Geometry: final body of the model. Coordinates: model frame, mm. Face numbers are marked on the shaded views. A direction names the side the tool comes from. Coordinates: 2 decimals unless noted, no trailing zeros. Write each loop counter-clockwise with the first axis right and the second up, starting at its lowest first coordinate (ties: lowest second). Pieces come first, ordered by that corner, then holes. Notation, with made-up numbers: M 12.25,-0.75 L 64.25,-0.75 A10 ccw 64.25,13.25 Z; hole C 58,84.5 d6. An arc over 180 degrees is marked long. Write item = value, one per line. Start each with the question number.
Item 1: Section C-C on x = 0. Output: boundary loops of the cut face in (y, z).
Item 2: Ray query, L1, parallel to X at y = -11.5, z = 0; L2, parallel to X at y = -4.5, z = 14; L3, parallel to Z at x = 0, y = -32.5. Return the intervals inside material, ascending. Write a range as [from, to].
Item 3: Reachability of the marked faces 4, 5, 6, 7 and 8 from +Z, -Z, +X, -X, +Y, -Y: full face, straight path, thin tool, end or side. Return the list, or none.
Item 4: Section A-A on z = 0. Output: boundary loops of the cut face in (x, y), plus the area to 3 significant figures.
Item 5: Section D-D on z = 19.5. Output: boundary loops of the cut face in (x, y).
Item 6: Pull-direction query (X, two-part tool) for the marked faces 1, 2 and 3; classes: +X half, -X half, draft (parallel to the pull), parting line (faces both ways), or undercut.
Item 7: Section B-B on y = -32.15. Output: boundary loops of the cut face in (x, z).
Item 8: First-contact query: pin 1 Ø5 at (x, z) = (-3.5, 13) entering from -Y; pin 2 Ø17 at (y, z) = (-13, 26.5) entering from +X; pin 3 Ø2 at (x, y) = (9.5, 6.5) entering from -Z; pin 4 Ø1.5 at (x, y) = (10, -40) entering from -Z. Flat tips, straight axial feed; report the tip coordinate or a pass-through.
from build123d import *

# Parameters (mm, degrees)
F0_R     = 13.25
F1_DEPTH = 50
F2_R     = 9.65
F3_DEPTH = 30.301
F5_DEPTH = 30.301
F7_DEPTH = 27.7
F8_W     = 11.7
F8_H     = 11.66135
F9_DEPTH = 50.001


with BuildPart() as f1:
    # F0 (on Front) → F1 (new body)
    with BuildSketch(Plane.XZ):
        with BuildLine():
            Line((-13.85, 42.55), (-13.85, 8.87581))
            ThreePointArc((-13.85, 8.87581), (0, -16.45), (13.85, 8.87581))
            Line((13.85, 8.87581), (13.85, 42.55))
            Line((13.85, 42.55), (-13.85, 42.55))
        make_face()
        Circle(F0_R, mode=Mode.SUBTRACT)
    extrude(amount=F1_DEPTH)

    # F2 (on face) → F3 (cut, through all)
    with BuildSketch(Plane(origin=(-13.85, 0, 0), x_dir=(0, -1, 0), z_dir=(-1, 0, 0))):
        with Locations((32.15, 27.4)):
            Circle(F2_R)
    extrude(amount=-F3_DEPTH, mode=Mode.SUBTRACT)

    # F4 (on face) → F5 (cut, through all)
    with BuildSketch(Plane(origin=(-13.85, 0, 0), x_dir=(0, -1, 0), z_dir=(-1, 0, 0))):
        Polygon((0, 23.55), (6, 30.757681), (0, 34.363233), align=None)
    extrude(amount=-F5_DEPTH, mode=Mode.SUBTRACT)

    # F6 (on face) → F7 (join)
    with BuildSketch(Plane(origin=(-13.85, 0, 0), x_dir=(0, -1, 0), z_dir=(-1, 0, 0))):
        Polygon((-14.600857, 42.55), (0, 34.363233), (0, 42.55), align=None)
    extrude(amount=-F7_DEPTH)

    # F8 (on face) → F9 (cut, through all)
    with BuildSketch(Plane(origin=(0, 0, 0), x_dir=(-1, 0, 0), z_dir=(0, 1, 0))):
        with Locations((0, 17.719325)):
            Rectangle(F8_W, F8_H)
        with BuildLine():
            ThreePointArc((13.25, 0), (11.248889, 7.001785), (5.85, 11.88865))
            Line((5.85, 11.88865), (-5.85, 11.88865))
            ThreePointArc((-5.85, 11.88865), (-7.001785, -11.248889), (13.25, 0))
        make_face()
    extrude(amount=-F9_DEPTH, mode=Mode.SUBTRACT)


solid = f1.part
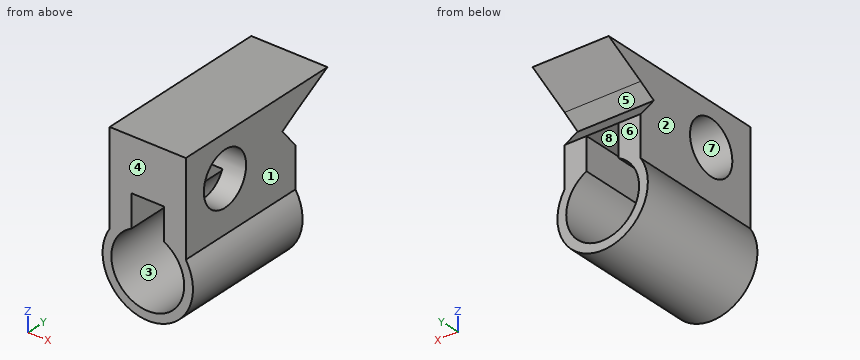
Responses:
q1.outline = M -50,-16.45 L 0,-16.45 L 0,-13.25 L -50,-13.25 Z; M -50,23.55 L -41,23.55 A9.65 cw long -23.3,23.55 L 0,23.55 L -6,30.76 L 0,34.36 L 14.6,42.55 L -50,42.55 Z
q2.L1 = [-16.45, -13.25], [13.25, 16.45]
q2.L2 = [-13.85, -5.85], [5.85, 13.85]
q2.L3 = [-16.45, -13.25], [37.04, 42.55]
q3.face_4 = +Z, -Z, +X, -X, -Y
q3.face_5 = +X, -X, +Y
q3.face_6 = -Z, +X, -X, +Y
q3.face_7 = +X, -X
q3.face_8 = +Y, -Y
q4.outline = M -16.45,-50 L -13.25,-50 L -13.25,0 L -16.45,0 Z; M 13.25,-50 L 16.45,-50 L 16.45,0 L 13.25,0 Z
q4.area = 320 mm²
q5.outline = M -13.85,-50 L -5.85,-50 L -5.85,-37.69 L -13.85,-37.69 Z; M -13.85,-26.61 L -5.85,-26.61 L -5.85,0 L -13.85,0 Z; M 5.85,-50 L 13.85,-50 L 13.85,-37.69 L 5.85,-37.69 Z; M 5.85,-26.61 L 13.85,-26.61 L 13.85,0 L 5.85,0 Z
q6.face_1 = +X half
q6.face_2 = -X half
q6.face_3 = undercut
q7.outline = M -13.85,8.88 A16.45 ccw long 13.85,8.88 L 13.85,17.75 L 5.85,17.75 L 5.85,11.89 A13.25 cw long -5.85,11.89 L -5.85,17.75 L -13.85,17.75 Z; M -13.85,37.05 L 13.85,37.05 L 13.85,42.55 L -13.85,42.55 Z
q8.pin_1 = -50
q8.pin_2 = 13.85
q8.pin_3 = 37.45
q8.pin_4 = -13.6
